from build123d import *

# Parameters (mm, degrees)
SKETCH1_W                = 598.17
SKETCH1_H                = 355.6
BOSS_EXTRUDE1_DEPTH      = 3.175
EDGE_FLANGE1_DEPTH       = 546.1
EDGE_FLANGE2_DEPTH       = 546.1
SKETCH13_R               = 2.0701
CUT_EXTRUDE1_DEPTH       = 474.928155862
LPATTERN1_COUNT          = 14
LPATTERN1_PITCH          = 25.4
MIRROR1_COPY_1_SKETCH_R  = 2.0701
MIRROR1_COPY_1_DEPTH     = 474.928155862
MIRROR1_COPY_2_SKETCH_R  = 2.0701
MIRROR1_COPY_2_DEPTH     = 474.928155862
MIRROR1_COPY_3_SKETCH_R  = 2.0701
MIRROR1_COPY_3_DEPTH     = 474.928155862
MIRROR1_COPY_4_SKETCH_R  = 2.0701
MIRROR1_COPY_4_DEPTH     = 474.928155862
MIRROR1_COPY_5_SKETCH_R  = 2.0701
MIRROR1_COPY_5_DEPTH     = 474.928155862
MIRROR1_COPY_6_SKETCH_R  = 2.0701
MIRROR1_COPY_6_DEPTH     = 474.928155862
MIRROR1_COPY_7_SKETCH_R  = 2.0701
MIRROR1_COPY_7_DEPTH     = 474.928155862
MIRROR1_COPY_8_SKETCH_R  = 2.0701
MIRROR1_COPY_8_DEPTH     = 474.928155862
MIRROR1_COPY_9_SKETCH_R  = 2.0701
MIRROR1_COPY_9_DEPTH     = 474.928155862
MIRROR1_COPY_10_SKETCH_R = 2.0701
MIRROR1_COPY_10_DEPTH    = 474.928155862
MIRROR1_COPY_11_SKETCH_R = 2.0701
MIRROR1_COPY_11_DEPTH    = 474.928155862
MIRROR1_COPY_12_SKETCH_R = 2.0701
MIRROR1_COPY_12_DEPTH    = 474.928155862
MIRROR1_COPY_13_SKETCH_R = 2.0701
MIRROR1_COPY_13_DEPTH    = 474.928155862
CUT_EXTRUDE2_START       = -224.492278251
CUT_EXTRUDE2_DEPTH       = 54.911587961
CUT_EXTRUDE2_START_2     = -134.630234215
CUT_EXTRUDE2_2_DEPTH     = 54.911587961
CUT_EXTRUDE2_START_3     = 109.584512833
CUT_EXTRUDE2_3_DEPTH     = 54.911587961
CUT_EXTRUDE2_START_4     = 217.879930564
CUT_EXTRUDE2_4_DEPTH     = 54.911587961


# Read off the part's stored shape, not the designer's step: Cut-Extrude2
# Sheet-metal steps are written as plain solids
with BuildPart() as part:
    # Sketch1 → Boss-Extrude1 (new body)
    with BuildSketch(Plane.XY.offset(370.818659046)):
        with Locations((0, 177.8)):
            Rectangle(SKETCH1_W, SKETCH1_H)
    extrude(amount=BOSS_EXTRUDE1_DEPTH)

    # Edge-Flange1 section (across the edge) → Edge-Flange1 (add)
    with BuildSketch(Plane(origin=(273.05, -1.315128061, 370.818659046), x_dir=(0, 0.7071067811865438, -0.7071067811865512), z_dir=(-1, 0, 0))):
        with BuildLine():
            Line((-3.175, 1.315128061), (-3.175, 20.509847662))
            Line((-3.175, 20.509847662), (0, 20.509847662))
            Line((0, 20.509847662), (0, 1.315128061))
            ThreePointArc((0, 1.315128061), (0.241682484, 0.100108163), (0.92993597, -0.92993597))
            Line((0.92993597, -0.92993597), (-1.315128061, -3.175))
            ThreePointArc((-1.315128061, -3.175), (-2.691635031, -1.114911735), (-3.175, 1.315128061))
        make_face()
    extrude(amount=EDGE_FLANGE1_DEPTH)

    # Edge-Flange2 section (across the edge) → Edge-Flange2 (add)
    with BuildSketch(Plane(origin=(-273.05, 356.915128061, 370.818659046), x_dir=(0, -0.7071067811865438, -0.7071067811865512), z_dir=(1, 0, 0))):
        with BuildLine():
            Line((-3.175, 1.315128061), (-3.175, 11.384871939))
            Line((-3.175, 11.384871939), (0, 11.384871939))
            Line((0, 11.384871939), (0, 1.315128061))
            ThreePointArc((0, 1.315128061), (0.241682484, 0.100108163), (0.92993597, -0.92993597))
            Line((0.92993597, -0.92993597), (-1.315128061, -3.175))
            ThreePointArc((-1.315128061, -3.175), (-2.691635031, -1.114911735), (-3.175, 1.315128061))
        make_face()
    extrude(amount=EDGE_FLANGE2_DEPTH)

    # Sketch13 → Cut-Extrude1 (cut, symmetric)
    with BuildSketch(Plane.XY.offset(373.993659046)):
        with Locations(Location((-288.925, 342.9, 0), (0, 0, 180))):
            Circle(SKETCH13_R)
    cut_extrude1 = extrude(amount=CUT_EXTRUDE1_DEPTH, both=True, mode=Mode.SUBTRACT)

    # LPattern1: Cut-Extrude1 ×14
    with Locations(*[(0, -i * LPATTERN1_PITCH, 0) for i in range(1, LPATTERN1_COUNT)]):
        add(cut_extrude1, mode=Mode.SUBTRACT)

    # Mirror1: Cut-Extrude1 across plane
    add(cut_extrude1.mirror(Plane.ZY), mode=Mode.SUBTRACT)

    # Mirror1 copy 1 sketch → Mirror1 copy 1 (cut, symmetric)
    with BuildSketch(Plane(origin=(0, -25.4, 373.993659046), x_dir=(-1, 0, 0), z_dir=(0, 0, 1))):
        with Locations((-288.925, -342.9)):
            Circle(MIRROR1_COPY_1_SKETCH_R)
    extrude(amount=MIRROR1_COPY_1_DEPTH, both=True, mode=Mode.SUBTRACT)

    # Mirror1 copy 2 sketch → Mirror1 copy 2 (cut, symmetric)
    with BuildSketch(Plane(origin=(0, -50.8, 373.993659046), x_dir=(-1, 0, 0), z_dir=(0, 0, 1))):
        with Locations((-288.925, -342.9)):
            Circle(MIRROR1_COPY_2_SKETCH_R)
    extrude(amount=MIRROR1_COPY_2_DEPTH, both=True, mode=Mode.SUBTRACT)

    # Mirror1 copy 3 sketch → Mirror1 copy 3 (cut, symmetric)
    with BuildSketch(Plane(origin=(0, -76.2, 373.993659046), x_dir=(-1, 0, 0), z_dir=(0, 0, 1))):
        with Locations((-288.925, -342.9)):
            Circle(MIRROR1_COPY_3_SKETCH_R)
    extrude(amount=MIRROR1_COPY_3_DEPTH, both=True, mode=Mode.SUBTRACT)

    # Mirror1 copy 4 sketch → Mirror1 copy 4 (cut, symmetric)
    with BuildSketch(Plane(origin=(0, -101.6, 373.993659046), x_dir=(-1, 0, 0), z_dir=(0, 0, 1))):
        with Locations((-288.925, -342.9)):
            Circle(MIRROR1_COPY_4_SKETCH_R)
    extrude(amount=MIRROR1_COPY_4_DEPTH, both=True, mode=Mode.SUBTRACT)

    # Mirror1 copy 5 sketch → Mirror1 copy 5 (cut, symmetric)
    with BuildSketch(Plane(origin=(0, -127, 373.993659046), x_dir=(-1, 0, 0), z_dir=(0, 0, 1))):
        with Locations((-288.925, -342.9)):
            Circle(MIRROR1_COPY_5_SKETCH_R)
    extrude(amount=MIRROR1_COPY_5_DEPTH, both=True, mode=Mode.SUBTRACT)

    # Mirror1 copy 6 sketch → Mirror1 copy 6 (cut, symmetric)
    with BuildSketch(Plane(origin=(0, -152.4, 373.993659046), x_dir=(-1, 0, 0), z_dir=(0, 0, 1))):
        with Locations((-288.925, -342.9)):
            Circle(MIRROR1_COPY_6_SKETCH_R)
    extrude(amount=MIRROR1_COPY_6_DEPTH, both=True, mode=Mode.SUBTRACT)

    # Mirror1 copy 7 sketch → Mirror1 copy 7 (cut, symmetric)
    with BuildSketch(Plane(origin=(0, -177.8, 373.993659046), x_dir=(-1, 0, 0), z_dir=(0, 0, 1))):
        with Locations((-288.925, -342.9)):
            Circle(MIRROR1_COPY_7_SKETCH_R)
    extrude(amount=MIRROR1_COPY_7_DEPTH, both=True, mode=Mode.SUBTRACT)

    # Mirror1 copy 8 sketch → Mirror1 copy 8 (cut, symmetric)
    with BuildSketch(Plane(origin=(0, -203.2, 373.993659046), x_dir=(-1, 0, 0), z_dir=(0, 0, 1))):
        with Locations((-288.925, -342.9)):
            Circle(MIRROR1_COPY_8_SKETCH_R)
    extrude(amount=MIRROR1_COPY_8_DEPTH, both=True, mode=Mode.SUBTRACT)

    # Mirror1 copy 9 sketch → Mirror1 copy 9 (cut, symmetric)
    with BuildSketch(Plane(origin=(0, -228.6, 373.993659046), x_dir=(-1, 0, 0), z_dir=(0, 0, 1))):
        with Locations((-288.925, -342.9)):
            Circle(MIRROR1_COPY_9_SKETCH_R)
    extrude(amount=MIRROR1_COPY_9_DEPTH, both=True, mode=Mode.SUBTRACT)

    # Mirror1 copy 10 sketch → Mirror1 copy 10 (cut, symmetric)
    with BuildSketch(Plane(origin=(0, -254, 373.993659046), x_dir=(-1, 0, 0), z_dir=(0, 0, 1))):
        with Locations((-288.925, -342.9)):
            Circle(MIRROR1_COPY_10_SKETCH_R)
    extrude(amount=MIRROR1_COPY_10_DEPTH, both=True, mode=Mode.SUBTRACT)

    # Mirror1 copy 11 sketch → Mirror1 copy 11 (cut, symmetric)
    with BuildSketch(Plane(origin=(0, -279.4, 373.993659046), x_dir=(-1, 0, 0), z_dir=(0, 0, 1))):
        with Locations((-288.925, -342.9)):
            Circle(MIRROR1_COPY_11_SKETCH_R)
    extrude(amount=MIRROR1_COPY_11_DEPTH, both=True, mode=Mode.SUBTRACT)

    # Mirror1 copy 12 sketch → Mirror1 copy 12 (cut, symmetric)
    with BuildSketch(Plane(origin=(0, -304.8, 373.993659046), x_dir=(-1, 0, 0), z_dir=(0, 0, 1))):
        with Locations((-288.925, -342.9)):
            Circle(MIRROR1_COPY_12_SKETCH_R)
    extrude(amount=MIRROR1_COPY_12_DEPTH, both=True, mode=Mode.SUBTRACT)

    # Mirror1 copy 13 sketch → Mirror1 copy 13 (cut, symmetric)
    with BuildSketch(Plane(origin=(0, -330.2, 373.993659046), x_dir=(-1, 0, 0), z_dir=(0, 0, 1))):
        with Locations((-288.925, -342.9)):
            Circle(MIRROR1_COPY_13_SKETCH_R)
    extrude(amount=MIRROR1_COPY_13_DEPTH, both=True, mode=Mode.SUBTRACT)

    # Cut-Extrude2 outline → Cut-Extrude2 (cut)
    with BuildSketch(Plane.YZ.offset(CUT_EXTRUDE2_START)):
        with BuildLine():
            Line((-4.490128061, 372.133787106), (-5.170256121, 371.453659046))
            Line((-5.170256121, 371.453659046), (-2.925192091, 369.208595015))
            Line((-2.925192091, 369.208595015), (-2.24506403, 369.888723076))
            ThreePointArc((-2.24506403, 369.888723076), (-1.215019898, 370.576976561), (0, 370.818659046))
            Line((0, 370.818659046), (56.283587678, 370.818659046))
            Line((56.283587678, 370.818659046), (56.283587678, 373.993659046))
            Line((56.283587678, 373.993659046), (0, 373.993659046))
            ThreePointArc((0, 373.993659046), (-2.430039796, 373.510294077), (-4.490128061, 372.133787106))
        make_face()
    extrude(amount=CUT_EXTRUDE2_DEPTH, mode=Mode.SUBTRACT)

    # Cut-Extrude2 2 outline → Cut-Extrude2 2 (cut)
    with BuildSketch(Plane.YZ.offset(CUT_EXTRUDE2_START_2)):
        with BuildLine():
            Line((-4.490128061, 372.133787106), (-5.170256121, 371.453659046))
            Line((-5.170256121, 371.453659046), (-2.925192091, 369.208595015))
            Line((-2.925192091, 369.208595015), (-2.24506403, 369.888723076))
            ThreePointArc((-2.24506403, 369.888723076), (-1.215019898, 370.576976561), (0, 370.818659046))
            Line((0, 370.818659046), (56.283587678, 370.818659046))
            Line((56.283587678, 370.818659046), (56.283587678, 373.993659046))
            Line((56.283587678, 373.993659046), (0, 373.993659046))
            ThreePointArc((0, 373.993659046), (-2.430039796, 373.510294077), (-4.490128061, 372.133787106))
        make_face()
    extrude(amount=CUT_EXTRUDE2_2_DEPTH, mode=Mode.SUBTRACT)

    # Cut-Extrude2 3 outline → Cut-Extrude2 3 (cut)
    with BuildSketch(Plane.YZ.offset(CUT_EXTRUDE2_START_3)):
        with BuildLine():
            Line((-4.490128061, 372.133787106), (-5.170256121, 371.453659046))
            Line((-5.170256121, 371.453659046), (-2.925192091, 369.208595015))
            Line((-2.925192091, 369.208595015), (-2.24506403, 369.888723076))
            ThreePointArc((-2.24506403, 369.888723076), (-1.215019898, 370.576976561), (0, 370.818659046))
            Line((0, 370.818659046), (56.283587678, 370.818659046))
            Line((56.283587678, 370.818659046), (56.283587678, 373.993659046))
            Line((56.283587678, 373.993659046), (0, 373.993659046))
            ThreePointArc((0, 373.993659046), (-2.430039796, 373.510294077), (-4.490128061, 372.133787106))
        make_face()
    extrude(amount=CUT_EXTRUDE2_3_DEPTH, mode=Mode.SUBTRACT)

    # Cut-Extrude2 4 outline → Cut-Extrude2 4 (cut)
    with BuildSketch(Plane.YZ.offset(CUT_EXTRUDE2_START_4)):
        with BuildLine():
            Line((-4.490128061, 372.133787106), (-5.170256121, 371.453659046))
            Line((-5.170256121, 371.453659046), (-2.925192091, 369.208595015))
            Line((-2.925192091, 369.208595015), (-2.24506403, 369.888723076))
            ThreePointArc((-2.24506403, 369.888723076), (-1.215019898, 370.576976561), (0, 370.818659046))
            Line((0, 370.818659046), (56.283587678, 370.818659046))
            Line((56.283587678, 370.818659046), (56.283587678, 373.993659046))
            Line((56.283587678, 373.993659046), (0, 373.993659046))
            ThreePointArc((0, 373.993659046), (-2.430039796, 373.510294077), (-4.490128061, 372.133787106))
        make_face()
    extrude(amount=CUT_EXTRUDE2_4_DEPTH, mode=Mode.SUBTRACT)


solid = part.part
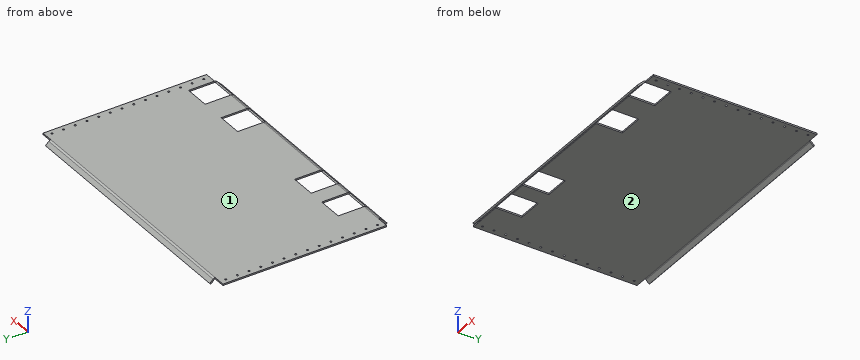
Design review of the part built by this model. Coordinates are the model's own, in mm. Face numbers are marked on the shaded views. Give positions to 0.01 mm unless a question says otherwise; leave off trailing zeros. Loops run counter-clockwise (first coordinate to the right, second up) from the corner with the lowest first, then second, coordinate; pieces in that order, holes last. Notation, with made-up numbers: M -35,79 L -11,79 A19 ccw -11,107 Z; hole C 52,21 d8. An arc over 180 degrees is marked long. Answer as a JSON object with one key per item and string values.
Item 1: Mouldability with a two-part tool opening along Y and no side actions: class the marked faces 1 and 2 as pulls with the +Y half, pulls with the -Y half, needs draft (parallel to the pull), parting line crosses it, or undercut.
Output values:
{"face 1": "needs draft", "face 2": "undercut"}
Item 2: Wall thickness on line 1 along X through (y, z) = (342.9, 373.1) (3 decimals); line 2 along Z through (x, y) = (106, 302.5); line 3 along Y through (x, z) = (-248.5, 367.75): over which ranges is each line inside the solid? List them lowest first.
Output values:
{"line 1": "x = -299.085 to -290.995, -286.855 to 286.855, 290.995 to 299.085", "line 2": "z = 370.82 to 373.99", "line 3": "y = -8.87 to -4.38, 359.98 to 364.47"}
Item 3: We need section C-C (y = 128.5). State the section outline as (x, z) points (3 decimals), and give its area (3 significant figures).
Output values:
{"outline": "M -299.085,370.819 L 299.085,370.819 L 299.085,373.994 L -299.085,373.994 Z", "area": "1,900 mm2"}
Item 4: We need section B-B (x = 204.5). State the section outline as (y, z) points (3 decimals), and give its area (3 significant figures).
Output values:
{"outline": "M -18.063,358.561 L -15.818,356.316 L -2.245,369.889 A3.175 cw 0,370.819 L 355.6,370.819 A3.175 cw 357.845,369.889 L 364.965,362.768 L 367.211,365.013 L 360.09,372.134 A6.35 ccw 355.6,373.994 L 0,373.994 A6.35 ccw -4.49,372.134 Z", "area": "1,250 mm2"}
Item 5: For P1, Ø6.5, axis at x = 288.925, y = 266.7, coming from the +Z side; P2, Ø2.5, axis at x = 282, z = 372.5, coming from the -Y side; P3, Ø8, axis at x = -139, y = 262, coming from the -Z side; P4, Ø2.5, axis at x = 245, z = 372.5, coming from the -Y side, all flat-tipped, find the tip position at first contact; note any pin that passes through.
Output values:
{"P1": "stops at z = 373.99", "P2": "stops at y = 0", "P3": "stops at z = 370.82", "P4": "stops at y = -5.37"}
Item 6: We need section A-A (x = -189.5). State the section outline as (y, z) points (3 decimals), and give its area (3 significant figures).
Output values:
{"outline": "M -18.063,358.561 L -15.818,356.316 L -2.925,369.209 L -5.17,371.454 Z; M 56.284,370.819 L 355.6,370.819 A3.175 cw 357.845,369.889 L 364.965,362.768 L 367.211,365.013 L 360.09,372.134 A6.35 ccw 355.6,373.994 L 56.284,373.994 Z", "area": "1,050 mm2"}
